from build123d import *

# Parameters (mm, degrees)
F1_DEPTH = 10
F2_R     = 4
F3_R     = 4.3
F5_D     = 4.3
F6_R     = 4
F7_DEPTH = 9


with BuildPart() as f1:
    # F0 (on Top) → F1 (new body)
    with BuildSketch(Plane.XY):
        Polygon((42.874504, 24.587632), (-16.125496, 24.587632), (-16.125496, -25.412368), (42.874504, -25.412368), (42.874504, -15.412368), (8.874504, -15.412368), (8.874504, 14.587632), (42.874504, 14.587632), align=None)
    extrude(amount=F1_DEPTH)

    # F2
    f2_edges = [f1.edges().sort_by_distance(p)[0] for p in [
        (8.874504, 14.587632, 5),
        (8.874504, -15.412368, 5),
    ]]
    fillet(f2_edges, radius=F2_R)

    # F3
    f3_edges = [f1.edges().sort_by_distance(p)[0] for p in [
        (-16.125496, 24.587632, 5),
        (-16.125496, -25.412368, 5),
    ]]
    fillet(f3_edges, radius=F3_R)

    # F5 (through all)
    with Locations(Plane.XY.offset(10)):
        with Locations((-11.825496, 20.287632), (-11.825496, -13.112368), (-11.825496, -21.112368)):
            Hole(F5_D / 2)

    # F6 (on face) → F7 (join)
    with BuildSketch(Plane(origin=(-16.125496, 0, 0), x_dir=(0, -1, 0), z_dir=(-1, 0, 0))):
        with Locations((-12.587632, 5)):
            Circle(F6_R)
    extrude(amount=F7_DEPTH)


solid = f1.part
Source: CAD feature listing. Evaluate the final solid. Frame: model axes, mm. A direction names the side the tool comes from. Give positions to 0.01 mm unless a question says otherwise; leave off trailing zeros. Write each loop counter-clockwise with the first axis right and the second up, starting at its lowest first coordinate (ties: lowest second). Pieces come first, ordered by that corner, then holes. Notation, with made-up numbers: M 51,83.25 L 93,83.25 A11 cw 93,91.25 Z; hole C 11,-11 d8. An arc over 180 degrees is marked long. Return JSON: item names as keys, results as strings. Group by question number.
1) Cut plane C-C, the plane y = -14.5. Output: boundary loops of the cut face in (x, z).
2) Material intervals for line 1 along X through (y, z) = (-21, 8.5); line 2 along Y through (x, z) = (34.5, 3.75); line 3 along X through (y, z) = (7, 3.5), sorted ascending. Write a range as [from, to].
3) Pull-direction query (X, two-part tool) for faces 1 (the face through (-10.12, -14.42, 4.93)), 2 (the face through (-14.83, -24.19, 5.07)), 3 (the face through (-11.36, 18.19, 4.93)), 4 (the face through (10.077, -14.272, 5.07)); classes: pulls with the +X half, pulls with the -X half, needs draft (parallel to the pull), parting line crosses it, or undercut.
4) Cut plane A-A, the plane x = 24. Output: boundary loops of the cut face in (y, z).
5) Set-up query: faces 5 (the face through (10.015, 13.385, 5.07)), 6 (the face through (42.875, 20, 5)), 7 (the face through (-20.562, 15.762, 2.566)). Return all of +Z, -Z, +X, -X, +Y, -Y with unobstructed straight access to the full face (end or side cutting, diameter ignored); none if empty.
6) Pin query (flat end, axial travel): P1, Ø5, axis at x = -11.83, y = -21.11, coming from the +Z side; P2, Ø3, axis at y = 6.5, z = 7.5, coming from the -X side; P3, Ø4, axis at y = 12, z = 3.5, coming from the +X side. Return the tip coordinate at first contact, or that it passes through.
7) Cut plane B-B, the plane z = 7.75. Output: boundary loops of the cut face in (x, y), plus the area to 3 significant figures.
8) Cut plane D-D, the plane x = -13. Output: boundary loops of the cut face in (y, z), plus the area to 3 significant figures.
Recorded:
{
 "1": {"outline": "M -16.13,0 L -13.47,0 L -13.47,10 L -16.13,10 Z; M -10.18,0 L 10.33,0 L 10.33,10 L -10.18,10 Z"},
 "2": {"line 1": "x = [-16.13, -13.97], [-9.68, 42.87]", "line 2": "y = [-25.41, -15.41], [14.59, 24.59]", "line 3": "x = [-16.13, 8.87]"},
 "3": {"face 1": "undercut", "face 2": "pulls with the -X half", "face 3": "undercut", "face 4": "pulls with the +X half"},
 "4": {"outline": "M -25.41,0 L -15.41,0 L -15.41,10 L -25.41,10 Z; M 14.59,0 L 24.59,0 L 24.59,10 L 14.59,10 Z"},
 "5": {"face 5": "+Z, -Z, +X", "face 6": "+Z, -Z, +X, +Y, -Y", "face 7": "-X"},
 "6": {"P1": "stops at z = 10", "P2": "stops at x = -16.13", "P3": "stops at x = 10.79"},
 "7": {"outline": "M -25.13,9.68 L -16.13,9.68 L -16.13,-21.11 A4.3 ccw -11.83,-25.41 L 42.87,-25.41 L 42.87,-15.41 L 12.87,-15.41 A4 cw 8.87,-11.41 L 8.87,10.59 A4 cw 12.87,14.59 L 42.87,14.59 L 42.87,24.59 L -11.83,24.59 A4.3 ccw -16.13,20.29 L -16.13,15.49 L -25.13,15.49 Z; hole C -11.83,-21.11 d4.3; hole C -11.83,-13.11 d4.3; hole C -11.83,20.29 d4.3", "area": "1,940 mm²"},
 "8": {"outline": "M -25.25,0 L -22.91,0 L -22.91,10 L -25.25,10 Z; M -19.31,0 L -14.91,0 L -14.91,10 L -19.31,10 Z; M -11.31,0 L 18.49,0 L 18.49,10 L -11.31,10 Z; M 22.09,0 L 24.42,0 L 24.42,10 L 22.09,10 Z", "area": "389 mm²"}
}
